Geometry check sheet. Reference: the model listing, model coordinates, mm. A direction names the side the tool comes from. Coordinates: 2 decimals unless noted, no trailing zeros. Loops run counter-clockwise (first coordinate to the right, second up) from the corner with the lowest first, then second, coordinate; pieces in that order, holes last. Notation, with made-up numbers: (17.5, 36.5) - (74.5, 36.5) arc R6 ccw to (74.5, 47.5) - close; hole circle Ø6 at (44.5, -15.5). An arc over 180 degrees is marked (long way). One line per item, written item: value.
from build123d import *

# Parameters (mm, degrees)
ESQUISSE1_W             = 219
ESQUISSE1_H             = 125
BOSS_EXTRU_1_DEPTH      = 19
ESQUISSE3_W             = 213.8
ESQUISSE3_H             = 119.8
ENL_V_MAT_EXTRU_1_DEPTH = 7.7
ESQUISSE4_R             = 4.75
ENL_V_MAT_EXTRU_2_DEPTH = 253.87744067
CONG_4_SIZE             = 5
CONG_5_SIZE             = 5


with BuildPart() as part:
    # Esquisse1 → Boss.-Extru.1 (new body)
    with BuildSketch(Plane.XY):
        with Locations((109.5, 62.5)):
            Rectangle(ESQUISSE1_W, ESQUISSE1_H)
    extrude(amount=BOSS_EXTRU_1_DEPTH)

    # Esquisse3 → Enlèv. mat.-Extru.1 (cut)
    with BuildSketch(Plane(origin=(0, 0, 0), x_dir=(-1, 0, 0), z_dir=(0, 0, -1))):
        with Locations((-109.5, 62.5)):
            Rectangle(ESQUISSE3_W, ESQUISSE3_H)
    extrude(amount=-ENL_V_MAT_EXTRU_1_DEPTH, mode=Mode.SUBTRACT)

    # Esquisse4 → Enlèv. mat.-Extru.2 (cut, through all)
    with BuildSketch(Plane.XY.offset(19)):
        with Locations((17.15, 57.15)):
            Circle(ESQUISSE4_R)
        with Locations((17.15, 37.65)):
            Circle(ESQUISSE4_R)
        with Locations((17.15, 18.15)):
            Circle(ESQUISSE4_R)
    extrude(amount=-ENL_V_MAT_EXTRU_2_DEPTH, mode=Mode.SUBTRACT)

    # Congé4
    # a fillet whose section is not a circle: 5 mm, written as the material it takes off along each edge
    with BuildSketch(Plane(origin=(219, 0, -12.5), x_dir=(-1, 0, 0), z_dir=(0, 0, 1))) as cong_4_piece_1:
        with BuildLine():
            add(Edge.make_bspline([(CONG_4_SIZE, 0), (CONG_4_SIZE * 0.831801948466, 0), (CONG_4_SIZE * 0.663603896932, 0), (CONG_4_SIZE * 0.292893218813, -CONG_4_SIZE * 0.0716919198361), (CONG_4_SIZE * 0.0716919198361, -CONG_4_SIZE * 0.292893218813), (0, -CONG_4_SIZE * 0.663603896932), (0, -CONG_4_SIZE * 0.831801948466), (0, -CONG_4_SIZE)], knots=[0, 0, 0, 0, 0, 0, 0.5, 0.5, 1, 1, 1, 1, 1, 1], degree=5))
            Line((0, -CONG_4_SIZE), (0, 0))
            Line((0, 0), (CONG_4_SIZE, 0))
        make_face()
    extrude(amount=44, mode=Mode.SUBTRACT)

    # Congé5
    # a fillet whose section is not a circle: 5 mm, written as the material it takes off along each edge
    with BuildSketch(Plane(origin=(0, 125, -12.5), x_dir=(0, -1, 0), z_dir=(0, 0, 1)), Plane(origin=(0, 0, -12.5), x_dir=(1, 0, 0), z_dir=(0, 0, 1)), Plane(origin=(219, 125, -12.5), x_dir=(-1, 0, 0), z_dir=(0, 0, 1))) as cong_5_piece_1:
        with BuildLine():
            add(Edge.make_bspline([(CONG_5_SIZE, 0), (CONG_5_SIZE * 0.831801948466, 0), (CONG_5_SIZE * 0.663603896932, 0), (CONG_5_SIZE * 0.292893218813, CONG_5_SIZE * 0.0716919198361), (CONG_5_SIZE * 0.0716919198361, CONG_5_SIZE * 0.292893218813), (0, CONG_5_SIZE * 0.663603896932), (0, CONG_5_SIZE * 0.831801948466), (0, CONG_5_SIZE)], knots=[0, 0, 0, 0, 0, 0, 0.5, 0.5, 1, 1, 1, 1, 1, 1], degree=5))
            Line((0, CONG_5_SIZE), (0, 0))
            Line((0, 0), (CONG_5_SIZE, 0))
        make_face()
    extrude(amount=44, mode=Mode.SUBTRACT)


solid = part.part
(1) Go/stop test with flat-tipped pins: pin 1 Ø15 at (x, y) = (17.15, 57.15) entering from -Z; pin 2 Ø8.5 at (x, y) = (17.15, 37.65) entering from +Z. Record where each tip stops, or that it passes through.
Reply:
pin 1: z = 7.7
pin 2: through
(2) Cross-section at B-B on y = 18.15. Record the cut outline in (x, z).
Reply:
outline: (0, 0) - (2.6, 0) - (2.6, 7.7) - (12.4, 7.7) - (12.4, 19) - (0, 19) - close; (21.9, 7.7) - (216.4, 7.7) - (216.4, 0) - (219, 0) - (219, 19) - (21.9, 19) - close
(3) Cross-section at A-A on x = 17.15. Record the cut outline in (y, z), and give its area (3 significant figures).
Reply:
outline: (0, 0) - (2.6, 0) - (2.6, 7.7) - (13.4, 7.7) - (13.4, 19) - (0, 19) - close; (22.9, 7.7) - (32.9, 7.7) - (32.9, 19) - (22.9, 19) - close; (42.4, 7.7) - (52.4, 7.7) - (52.4, 19) - (42.4, 19) - close; (61.9, 7.7) - (122.4, 7.7) - (122.4, 0) - (125, 0) - (125, 19) - (61.9, 19) - close
area: 1,130 mm2
(4) Cross-section at C-C on y = 71.5. Record the cut outline in (x, z), and give its area (3 significant figures).
Reply:
outline: (0, 0) - (2.6, 0) - (2.6, 7.7) - (216.4, 7.7) - (216.4, 0) - (219, 0) - (219, 19) - (0, 19) - close
area: 2,510 mm2
(5) Material ranges on probe 1 along Y at (x, z) = (17.15, 10.75); probe 2 along X at (y, z) = (17.5, 15); probe 3 along Y at (x, z) = (201, 1), recorded low to high. Write a range as from..to.
Reply:
probe 1: 0..13.4, 22.9..32.9, 42.4..52.4, 61.9..125
probe 2: 0..12.44, 21.86..219
probe 3: 0..2.6, 122.4..125
(6) Cross-section at D-D on x = 96.5. Record the cut outline in (y, z), and give its area (3 significant figures).
Reply:
outline: (0, 0) - (2.6, 0) - (2.6, 7.7) - (122.4, 7.7) - (122.4, 0) - (125, 0) - (125, 19) - (0, 19) - close
area: 1,450 mm2
(7) Access from +Z, -Z, +X, -X, +Y, -Y to the whole of each face (thin tool, end or side, straight path). Record for faces 1 (the face through (111, 2.6, 4)), 2 (the face through (13.65, 40.86, 13.43)).
Reply:
face 1: -Z
face 2: +Z, -Z
(8) Release check for a two-part mould opening along Y. For faces 3 (the face through (219, 62, 9)), 4 (the face through (108, 0, 9)), 5 (the face through (16.53, 61.86, 13.43)) record: pulls with the +Y half, pulls with the -Y half, needs draft (parallel to the pull), parting line crosses it, or undercut.
Reply:
face 3: needs draft
face 4: pulls with the -Y half
face 5: undercut
